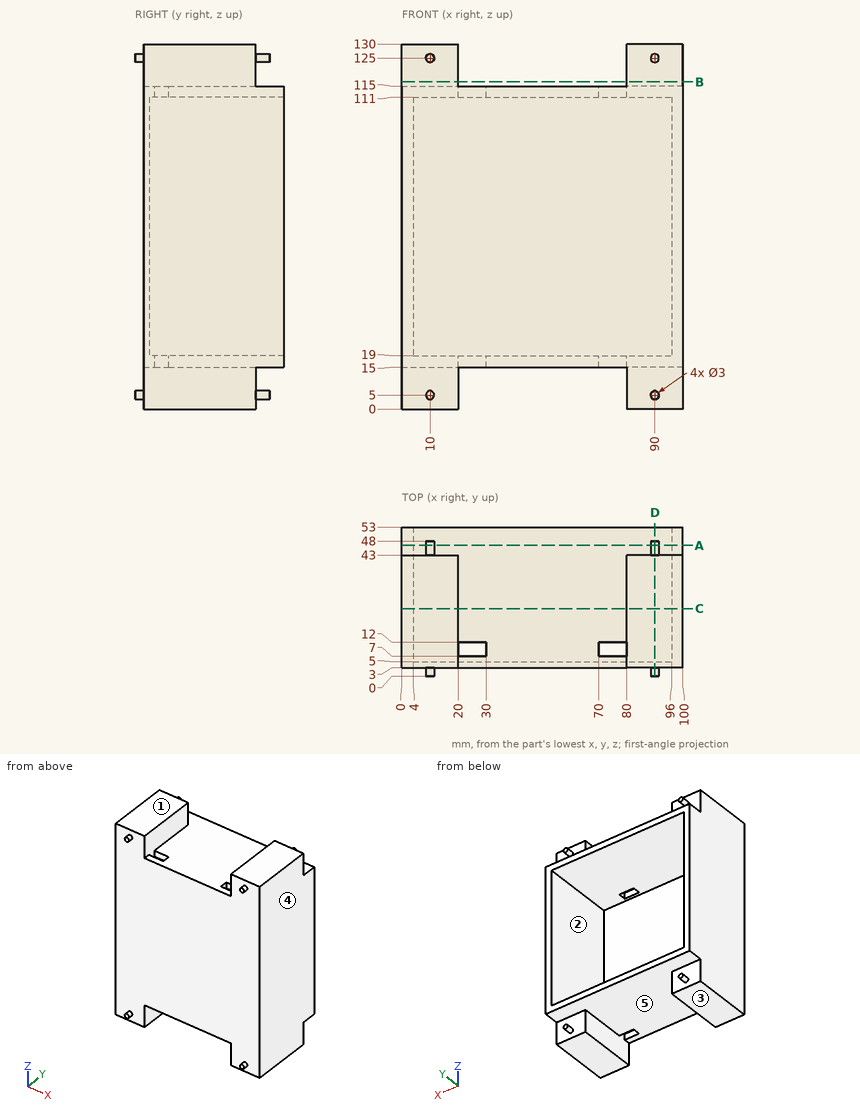
Input: dimensioned drawing with shaded views. Units: mm. Origin: part minimum x, y, z. A direction names the side the tool comes from. Round coordinates to 2 decimals unless told otherwise and drop trailing zeros. Order: outer loops, then holes, each group sorted by start corner. A loop starts at its lowest first (then second) coordinate and runs counter-clockwise, first axis right, second up. Notation, with made-up numbers: (-27.75, 82) - (20.25, 82) arc R23 ccw to (20.25, 117) - close; hole circle Ø4 at (-33, 52). An arc over 180 degrees is marked (long way). Write item = value, one per line. Start each with the question number.
Q1. Cut plane C-C on y = 24. Return the cut outline in (x, z).
Q2. Ray query, line 1 (Z direction, x = 67, y = 35); line 2 (X direction, y = 17, z = 66.5); line 3 (X direction, y = 35.5, z = 117). Return the intervals inside material, ascending. Write a range as from..to.
Q3. Cut plane D-D on x = 90. Return the cut outline in (y, z).
Q4. Cut plane A-A on y = 46.5. Return the cut outline in (x, z).
Q5. Cut plane B-B on z = 116.5. Return the cut outline in (x, y), and give its area (3 significant figures).
Q6. Pull-direction query (X, two-part tool) for the marked faces 3, 4 and 5; classes: +X half, -X half, draft (parallel to the pull), parting line (faces both ways), or undercut.
Q7. Pin query (flat end, axial travel): pin 1 (5 mm diameter, centred on x = 79, z = 76.5, fed in from +Y); pin 2 (3 mm diameter, centred on x = 31, z = 63, fed in from -Y); pin 3 (25 mm diameter, centred on x = 59, y = 24, fed in from -Z). Return the tip coordinate at first contact, or that it passes through.
Q8. Access query for the marked faces 1 and 2. Directions: +Z, -Z, +X, -X, +Y, -Y. A direction counts if a zero-diameter tool reaches every point of the face in a straight line with its end or side. Return the directions, or none.
Outcome:
q1.outline = (0, 0) - (20, 0) - (20, 15) - (80, 15) - (80, 0) - (100, 0) - (100, 130) - (80, 130) - (80, 115) - (20, 115) - (20, 130) - (0, 130) - close; hole (4, 19) - (96, 19) - (96, 111) - (4, 111) - close
q2.line_1 = 15..19, 111..115
q2.line_2 = 0..4, 96..100
q2.line_3 = 0..20, 80..100
q3.outline = (0, 3.5) - (3, 3.5) - (3, 0) - (43, 0) - (43, 3.5) - (48, 3.5) - (48, 6.5) - (43, 6.5) - (43, 15) - (53, 15) - (53, 19) - (5, 19) - (5, 111) - (53, 111) - (53, 115) - (43, 115) - (43, 123.5) - (48, 123.5) - (48, 126.5) - (43, 126.5) - (43, 130) - (3, 130) - (3, 126.5) - (0, 126.5) - (0, 123.5) - (3, 123.5) - (3, 6.5) - (0, 6.5) - close
q4.outline = (0, 15) - (100, 15) - (100, 115) - (0, 115) - close; circle Ø3 at (10, 5); circle Ø3 at (10, 125); circle Ø3 at (90, 5); circle Ø3 at (90, 125); hole (4, 19) - (96, 19) - (96, 111) - (4, 111) - close
q5.outline = (0, 3) - (20, 3) - (20, 43) - (0, 43) - close; (80, 3) - (100, 3) - (100, 43) - (80, 43) - close
q5.area = 1,600 mm^2
q6.face_3 = draft
q6.face_4 = +X half
q6.face_5 = undercut
q7.pin_1 = 5
q7.pin_2 = 3
q7.pin_3 = 15
q8.face_1 = +Z, +X, -X, +Y, -Y
q8.face_2 = +Y
